Work out the finished part from the listing and answer in its coordinate system (mm). A direction names the side the tool comes from. Coordinates: 2 decimals unless noted, no trailing zeros. Loops run counter-clockwise (first coordinate to the right, second up) from the corner with the lowest first, then second, coordinate; pieces in that order, holes last.
```python
from build123d import *

# Parameters (mm, degrees)
SKETCH1_R           = 75
BOSS_EXTRUDE1_DEPTH = 250
SKETCH2_R           = 12.5
CUT_EXTRUDE1_DEPTH  = 250


with BuildPart() as part:
    # Sketch1 → Boss-Extrude1 (new body)
    with BuildSketch(Plane.XY):
        with BuildLine():
            Line((325, 0), (-325, 0))
            Line((-325, 0), (-325, -32))
            Line((-325, -32), (-106, -32))
            Line((-106, -32), (-106, -132))
            ThreePointArc((-106, -132), (0, -238), (106, -132))
            Line((106, -132), (106, -32))
            Line((106, -32), (325, -32))
            Line((325, -32), (325, 0))
        make_face()
        with Locations((0, -132)):
            Circle(SKETCH1_R, mode=Mode.SUBTRACT)
    extrude(amount=BOSS_EXTRUDE1_DEPTH)

    # Sketch2 → Cut-Extrude1 (cut)
    with BuildSketch(Plane(origin=(0, 0, 0), x_dir=(1, 0, 0), z_dir=(0, 1, 0))):
        with Locations(Location((-250, -187.5, 0), (0, 0, 180))):  # turned: the seam where the file's is
            Circle(SKETCH2_R)
        with Locations(Location((-250, -62.5, 0), (0, 0, 180))):  # turned: the seam where the file's is
            Circle(SKETCH2_R)
        with Locations(Location((250, -187.5, 0), (0, 0, 90))):  # turned: the seam where the file's is
            Circle(SKETCH2_R)
        with Locations(Location((250, -62.5, 0), (0, 0, 90))):  # turned: the seam where the file's is
            Circle(SKETCH2_R)
    extrude(amount=-CUT_EXTRUDE1_DEPTH, mode=Mode.SUBTRACT)


solid = part.part
```
1. A cutting plane is placed at C-C, the plane y = -109.5. Give the vertices of the cut face in (x, z).
2. A cutting plane is placed at D-D, the plane z = 18. Give the vertices of the cut face in (x, y), then the cut area to 3 significant figures.
3. A cutting plane is placed at A-A, the plane z = 187.5. Give the vertices of the cut face in (x, y).
4. Determine the mould class of faces 4 (the flat face through (-1.5, -56.7, 250)), 5 (the cylindrical face through (-9.764, -57.638, 123.25)), 6 (the cylindrical face through (237.606, -15.776, 64.127)) for opening direction Z: released by +Z, released by -Z, zero draft, split by the parting line, or undercut.
5. For faces 1 (the flat face through (-106, -81, 123)), 2 (the flat face through (-325, -16, 123)), 3 (the flat face through (214, -32, 123)), determine the directions among +Z, -Z, +X, -X, +Y, -Y from which every point of the face is accessible in a straight line to the end or side of a thin tool.
6. A cutting plane is placed at B-B, the plane x = 0. Give the vertices of the cut face in (y, z).
7. Straight lines are drawn through the part: probe 1 along X at (y, z) = (-16, 187); probe 2 along Z at (x, y) = (250, -18); probe 3 along X at (y, z) = (-10, 189). For each, find the intervals that lie inside material, in ascending order.
8. Each of these flat-tipped pins is pushed along its axis until it touches: P1, Ø8, axis at y = -105.5, z = 175, coming from the -X side; P2, Ø22.5, axis at x = -250, z = 187.5, coming from the +Y side; P3, Ø1, axis at x = -240.5, z = 105, coming from the -Y side; P4, Ø6, axis at y = -128, z = 205.5, coming from the +X side. Where does it stop, or does it pass through?
Answers below:
1. outline: (-106, 0) - (-71.55, 0) - (-71.55, 250) - (-106, 250) - close; (71.55, 0) - (106, 0) - (106, 250) - (71.55, 250) - close
2. outline: (-325, -32) - (-106, -32) - (-106, -132) arc R106 ccw to (106, -132) - (106, -32) - (325, -32) - (325, 0) - (-325, 0) - close; hole circle Ø150 at (0, -132)
2. area: 42,000 mm2
3. outline: (-325, -32) - (-262.5, -32) - (-262.5, 0) - (-325, 0) - close; (-237.5, -32) - (-106, -32) - (-106, -132) arc R106 ccw to (106, -132) - (106, -32) - (237.5, -32) - (237.5, 0) - (-237.5, 0) - close; (262.5, -32) - (325, -32) - (325, 0) - (262.5, 0) - close; hole circle Ø150 at (0, -132)
4. face 4: released by +Z
4. face 5: zero draft
4. face 6: undercut
5. face 1: +Z, -Z, -X, -Y
5. face 2: +Z, -Z, -X, +Y, -Y
5. face 3: +Z, -Z, +X, -Y
6. outline: (-238, 0) - (-207, 0) - (-207, 250) - (-238, 250) - close; (-57, 0) - (0, 0) - (0, 250) - (-57, 250) - close
7. probe 1: x = -325 to -262.49, -237.51 to 237.51, 262.49 to 325
7. probe 2: z = 0 to 50, 75 to 175, 200 to 250
7. probe 3: x = -325 to -262.41, -237.59 to 237.59, 262.41 to 325
8. P1: stops at x = -106
8. P2: passes through
8. P3: stops at y = -32
8. P4: stops at x = 106
